Model file for the job. Use its own axes, mm. Give positions to 0.01 mm unless a question says otherwise; leave off trailing zeros. Write each loop counter-clockwise with the first axis right and the second up, starting at its lowest first coordinate (ties: lowest second). Pieces come first, ordered by that corner, then holes. Notation, with made-up numbers: (8.25, 14.5) - (20.25, 14.5) arc R36 ccw to (20.25, 48.5) - close; hole circle Ø3 at (17, 16). An arc over 180 degrees is marked (long way). Use CSV: the item, a comma, the result in double quotes.
from build123d import *

# Parameters (mm, degrees)
SKETCH2_W               = 3.87532504
SKETCH2_H               = 22.790076604
CUT_EXTRUDE1_DEPTH      = 21.133554083
CUT_EXTRUDE2_DEPTH      = 21.133554083
CUT_EXTRUDE2_DEPTH_BACK = 21.133554083


with BuildPart() as part:
    # Sketch1 → Revolve1 (revolve)
    with BuildSketch(Plane(origin=(0, 0, 0), x_dir=(0, 0, -1), z_dir=(1, 0, 0)), mode=Mode.PRIVATE) as revolve1_sk:
        Polygon((0, 0), (15.6, 0), (15.6, 7.25), (15.131088913, 9), (3.5, 9), (0, 7.72610418), align=None)
    revolve(revolve1_sk.sketch.rotate(Axis((0, 0, 0), (0, 0, -1)), 97.645107459), axis=Axis((0, 0, 0), (0, 0, -1)))

    # Sketch2 → Cut-Extrude1 (cut, through all)
    with BuildSketch(Plane.XY):
        with Locations((10.85766252, -0.726684939)):
            Rectangle(SKETCH2_W, SKETCH2_H)
    extrude(amount=-CUT_EXTRUDE1_DEPTH, mode=Mode.SUBTRACT)

    # Sketch3 → Cut-Extrude2 (cut, two sides: drawn at the far end of the back side and taken through both)
    with BuildSketch(Plane(origin=(0, 0, 0), x_dir=(0, 0, -1), z_dir=(1, 0, 0)).offset(-CUT_EXTRUDE2_DEPTH_BACK)):
        with BuildLine():
            Line((15.070887618, 0.152741588), (15.6, 0.6))
            Line((15.6, 0.6), (15.6, -0.6))
            Line((15.6, -0.6), (15.070887618, -0.152741588))
            ThreePointArc((15.070887618, -0.152741588), (15, 0), (15.070887618, 0.152741588))
        make_face()
    extrude(amount=CUT_EXTRUDE2_DEPTH + CUT_EXTRUDE2_DEPTH_BACK, mode=Mode.SUBTRACT)


solid = part.part
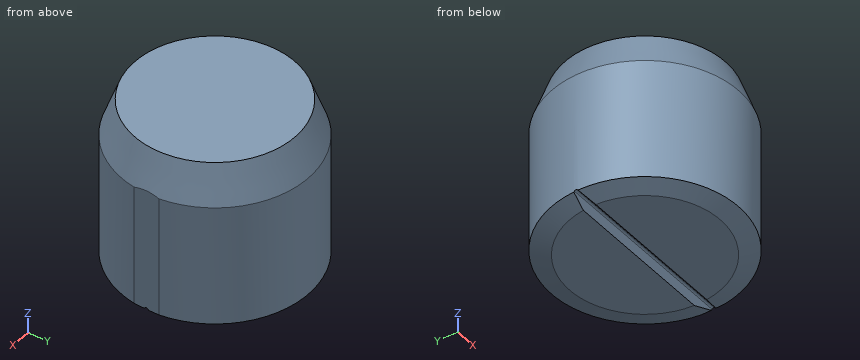
(1) Saw through at A-A, the plane x = 0. List the corners of the cut face in (y, z), then the cut area to 3 significant figures.
Checked values:
outline,"(-9, -15.13) - (-7.25, -15.6) - (-0.6, -15.6) - (-0.15, -15.07) arc R0.2 cw to (0.15, -15.07) - (0.6, -15.6) - (7.25, -15.6) - (9, -15.13) - (9, -3.5) - (7.73, 0) - (-7.73, 0) - (-9, -3.5) - close"
area,"275 mm^2"
(2) Saw through at B-B, the plane z = -5.75. List the corners of the cut face in (x, y).
Checked values:
outline,"(8.92, -1.2) - (8.92, 1.2) arc R9 ccw (long way) to start"
(3) Flat gauge pins, fed straight in: P1, Ø4, axis at y = -4, z = -11, coming from the +X side; P2, Ø5, axis at x = 3, z = -6.5, coming from the -Y side. Where does each tip first touch, or does it go through?
Checked values:
P1,"stops at x = 8.77"
P2,"stops at y = -8.99"
(4) Wall check: probe 1 along X at (y, z) = (3.75, -13.25); probe 2 along Y at (x, z) = (3.5, -1.5); probe 3 along X at (y, z) = (2, -3.25). Give the ranges that are in metal, low to high. Write a range as [from, to].
Checked values:
probe 1,"x = [-8.18, 8.18]"
probe 2,"y = [-7.5, 7.5]"
probe 3,"x = [-8.68, 8.68]"
